Study the drawing (mm; zero at the part's minimum x, y, z) and answer. Give positions to 0.01 mm unless a question says otherwise; leave off trailing zeros. Order: outer loops, then holes, each group sorted by start corner. A loop starts at its lowest first (then second) coordinate and runs counter-clockwise, first axis right, second up. Notation, with made-up numbers: (11.5, 16.25) -> (64.5, 16.25) arc R13 cw to (64.5, 40.25) -> close; hole circle Ø2 at (35.5, -24). An arc over 180 degrees is marked (long way). Use a Markdown table: item, result. Add a question column.
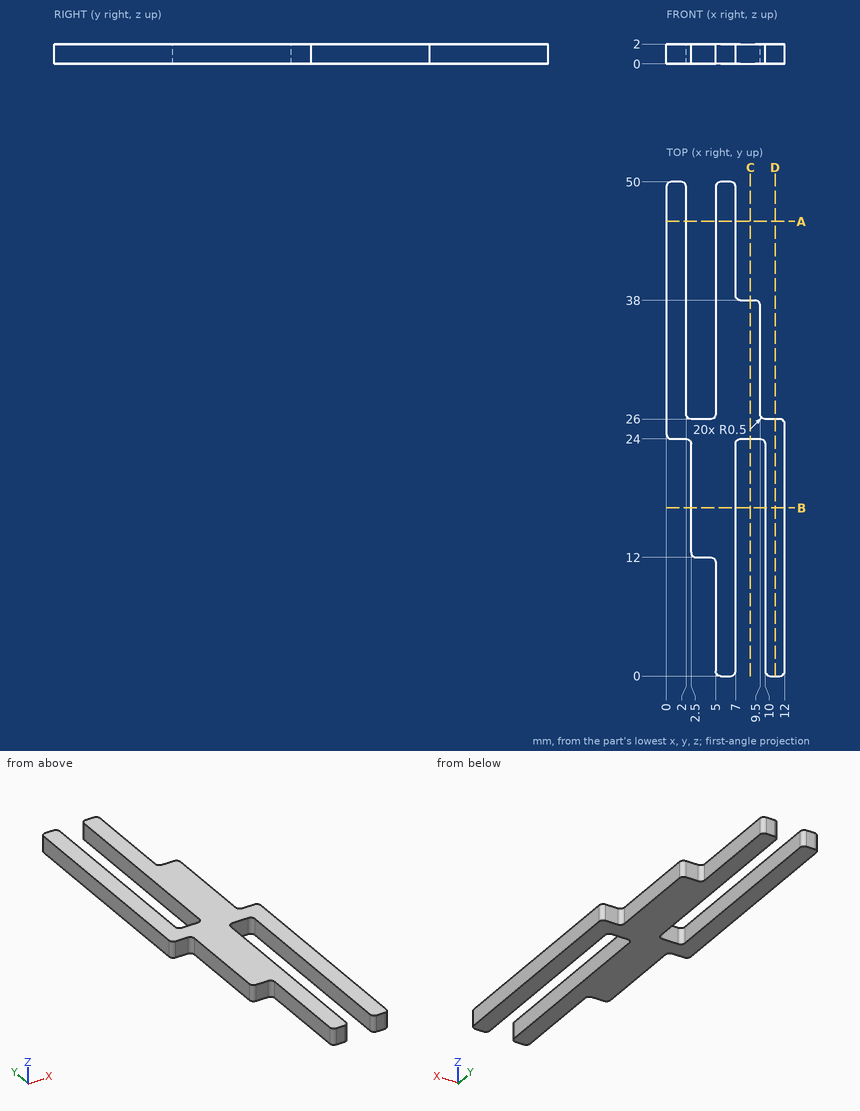
1) The part is cut by section B-B, the plane y = 17. Determine the outline of the cut face in (x, z).
2) Straight lines are drawn through the part: line 1 (X direction, y = 6.5, z = 0.6); line 2 (X direction, y = 20, z = 1.5); line 3 (Y direction, x = 11, z = 1.85). For each, find the intervals that lie inside material, in ascending order.
3) The part is cut by section A-A, the plane y = 46. Determine the outline of the cut face in (x, z).
4) A flat-ended cylindrical pin translates along its axis: pin 1 (0.8 mm diameter, centred on x = 8, z = 1, fed in from +Y). Find the tip coordinate at first contact, or state that the pin passes through.
5) The part is cut by section D-D, the plane x = 11. Determine the outline of the cut face in (y, z), then the cut area to 3 significant figures.
6) The part is cut by section C-C, the plane x = 8.5. Determine the outline of the cut face in (y, z).
A:
| question | item | result |
|---|---|---|
| 1 | outline | (2.5, 0) -> (7, 0) -> (7, 2) -> (2.5, 2) -> close; (10, 0) -> (12, 0) -> (12, 2) -> (10, 2) -> close |
| 2 | line 1 | 5 to 7, 10 to 12 |
| 2 | line 2 | 2.5 to 7, 10 to 12 |
| 2 | line 3 | 0 to 26 |
| 3 | outline | (0, 0) -> (2, 0) -> (2, 2) -> (0, 2) -> close; (5, 0) -> (7, 0) -> (7, 2) -> (5, 2) -> close |
| 4 | pin 1 | y = 38 |
| 5 | outline | (0, 0) -> (26, 0) -> (26, 2) -> (0, 2) -> close |
| 5 | area | 52.0 mm^2 |
| 6 | outline | (24, 0) -> (38, 0) -> (38, 2) -> (24, 2) -> close |
